```python
from build123d import *

# Parameters (mm, degrees)
BOSS_EXTRUDE1_DEPTH = 2


with BuildPart() as part:
    # Sketch1 → Boss-Extrude1 (new body)
    with BuildSketch(Plane(origin=(0, 0, 0), x_dir=(1, 0, 0), z_dir=(0, 1, 0))):
        with BuildLine():
            Line((-50.830454799, 13.264128767), (0, 17.5))
            Line((0, 17.5), (50.830454799, 13.264128767))
            ThreePointArc((50.830454799, 13.264128767), (57.358822867, 10.069766074), (60, 3.298671184))
            Line((60, 3.298671184), (60, -7.5))
            ThreePointArc((60, -7.5), (57.071067812, -14.571067812), (50, -17.5))
            Line((50, -17.5), (9.470954357, -17.5))
            Line((9.470954357, -17.5), (0, -7.5))
            Line((0, -7.5), (-10.529045643, -17.5))
            Line((-10.529045643, -17.5), (-50, -17.5))
            ThreePointArc((-50, -17.5), (-57.071067812, -14.571067812), (-60, -7.5))
            Line((-60, -7.5), (-60, 3.298671184))
            ThreePointArc((-60, 3.298671184), (-57.358822867, 10.069766074), (-50.830454799, 13.264128767))
        make_face()
    extrude(amount=BOSS_EXTRUDE1_DEPTH)


solid = part.part
```
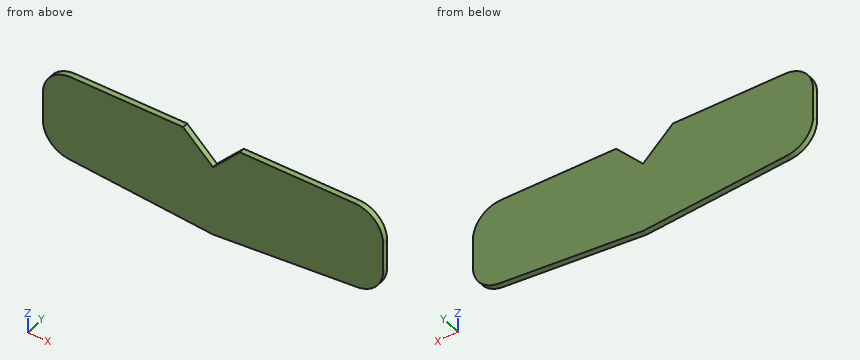
Model file for the job. Use its own axes, mm. Coordinates: 2 decimals unless noted, no trailing zeros. Order: outer loops, then holes, each group sorted by start corner. A loop starts at its lowest first (then second) coordinate and runs counter-clockwise, first axis right, second up. Notation, with made-up numbers: (12, 15.5) - (55, 15.5) arc R32 ccw to (55, 46.5) - close; hole circle Ø8 at (9, 60.25). An arc over 180 degrees is marked (long way). Return JSON: item names as keys, results as strings. Group by question number.
1) Probe line 1 (X direction, y = 1.2, z = 14); line 2 (X direction, y = 1.85, z = 15); line 3 (Z direction, x = 19.5, y = 1.5) (3 decimals). List the from-to ranges inside material, lowest first. Write a range as from..to.
2) Saw through at D-D, the plane z = -8.5. Write the cut outline in (x, y).
3) Saw through at A-A, the plane z = 12.5. Write the cut outline in (x, y), plus the area to 3 significant figures.
4) Saw through at B-B, the plane y = 1.05. Write the cut outline in (x, z).
5) Saw through at C-C, the plane x = 7.5. Write the cut outline in (y, z) (3 decimals), plus the area to 3 significant figures.
Values found:
{
 "1": {"line 1": "x = -57.6..-6.84, 6.16..57.6", "line 2": "x = -56.61..-7.9, 7.1..56.61", "line 3": "z = -15.875..17.5"},
 "2": {"outline": "(-58.54, 0) - (58.54, 0) - (58.54, 2) - (-58.54, 2) - close"},
 "3": {"outline": "(-58.66, 0) - (-5.26, 0) - (-5.26, 2) - (-58.66, 2) - close; (4.74, 0) - (58.66, 0) - (58.66, 2) - (4.74, 2) - close", "area": "215 mm²"},
 "4": {"outline": "(-60, -3.3) arc R10 ccw to (-50.83, -13.26) - (0, -17.5) - (50.83, -13.26) arc R10 ccw to (60, -3.3) - (60, 7.5) arc R10 ccw to (50, 17.5) - (9.47, 17.5) - (0, 7.5) - (-10.53, 17.5) - (-50, 17.5) arc R10 ccw to (-60, 7.5) - close"},
 "5": {"outline": "(0, -16.875) - (2, -16.875) - (2, 15.419) - (0, 15.419) - close", "area": "64.6 mm²"}
}
